Check sheet for the modelled part. Datum: model origin and axes. Units: mm. Give positions to 0.01 mm unless a question says otherwise; leave off trailing zeros. Order: outer loops, then holes, each group sorted by start corner. A loop starts at its lowest first (then second) coordinate and runs counter-clockwise, first axis right, second up.
```python
from build123d import *

# Parameters (mm, degrees)
SKETCH_1_W      = 330
SKETCH_1_H      = 30
SKETCH_1_R      = 3.25
SKETCH_1_R_2    = 1.75
EXTRUDE_1_DEPTH = 3
CHAMFER_1_SIZE  = 1.5


with BuildPart() as part:
    # Эскиз1 → Вытянуть1 (new body)
    with BuildSketch(Plane.XY):
        Rectangle(SKETCH_1_W, SKETCH_1_H)
        with Locations((135, 0)):
            Circle(SKETCH_1_R, mode=Mode.SUBTRACT)
        with Locations((90, 0)):
            Circle(SKETCH_1_R_2, mode=Mode.SUBTRACT)
        with Locations((45, 0)):
            Circle(SKETCH_1_R, mode=Mode.SUBTRACT)
        with Locations(Location((-45, 0, 0), (0, 0, 180))):
            Circle(SKETCH_1_R, mode=Mode.SUBTRACT)
        with Locations(Location((-90, 0, 0), (0, 0, 180))):
            Circle(SKETCH_1_R_2, mode=Mode.SUBTRACT)
        with Locations(Location((-135, 0, 0), (0, 0, 180))):
            Circle(SKETCH_1_R, mode=Mode.SUBTRACT)
    extrude(amount=EXTRUDE_1_DEPTH)

    # Фаска1
    chamfer_1_edges = [part.edges().sort_by_distance(p)[0] for p in [
        (88.25, 0, 3),
        (-88.25, 0, 3),
    ]]
    chamfer(chamfer_1_edges, length=CHAMFER_1_SIZE)


solid = part.part
```
(1) Cross-section at A-A on x = 135. Enter the section's corners in (y, z).
Response values:
outline: (-15, 0) - (-3.25, 0) - (-3.25, 3) - (-15, 3) - close; (3.25, 0) - (15, 0) - (15, 3) - (3.25, 3) - close
(2) Material ranges on L1, parallel to Y at x = -135, z = 0.95; L2, parallel to Y at x = -90, z = 0.7, recorded low to high.
Response values:
L1: y = -15 to -3.25, 3.25 to 15
L2: y = -15 to -1.75, 1.75 to 15
(3) Gauge pin test, flat ends, axial feed: pin 1 Ø2 at (x, y) = (63.5, -6.5) entering from -Z; pin 2 Ø5 at (x, y) = (45, 0) entering from +Z; pin 3 Ø5.5 at (x, y) = (90, 0) entering from +Z. Record the tip position at first contact, or that the pin passes through.
Response values:
pin 1: stops at z = 0
pin 2: passes through
pin 3: stops at z = 2.5
(4) Release check for a two-part mould opening along X. For faces 1 (the face through (48.002, -1.245, 1.479)), 2 (the face through (-2, 0, 3)) record: released by +X, released by -X, zero draft, split by the parting line, or undercut.
Response values:
face 1: undercut
face 2: zero draft
